Geometry: see drawing. Coordinates: mm, zero at the bounding-box minimum. A direction names the side the tool comes from. Coordinates: 2 decimals unless noted, no trailing zeros. Write each loop counter-clockwise with the first axis right and the second up, starting at its lowest first coordinate (ties: lowest second). Pieces come first, ordered by that corner, then holes. Notation, with made-up numbers: (-1.5, 39) -> (55.5, 39) arc R18 ccw to (55.5, 47) -> close; hole circle Ø1 at (29.25, 68.5). An arc over 180 degrees is marked (long way). Answer as a JSON object with one key per item and string values. Group by question number.
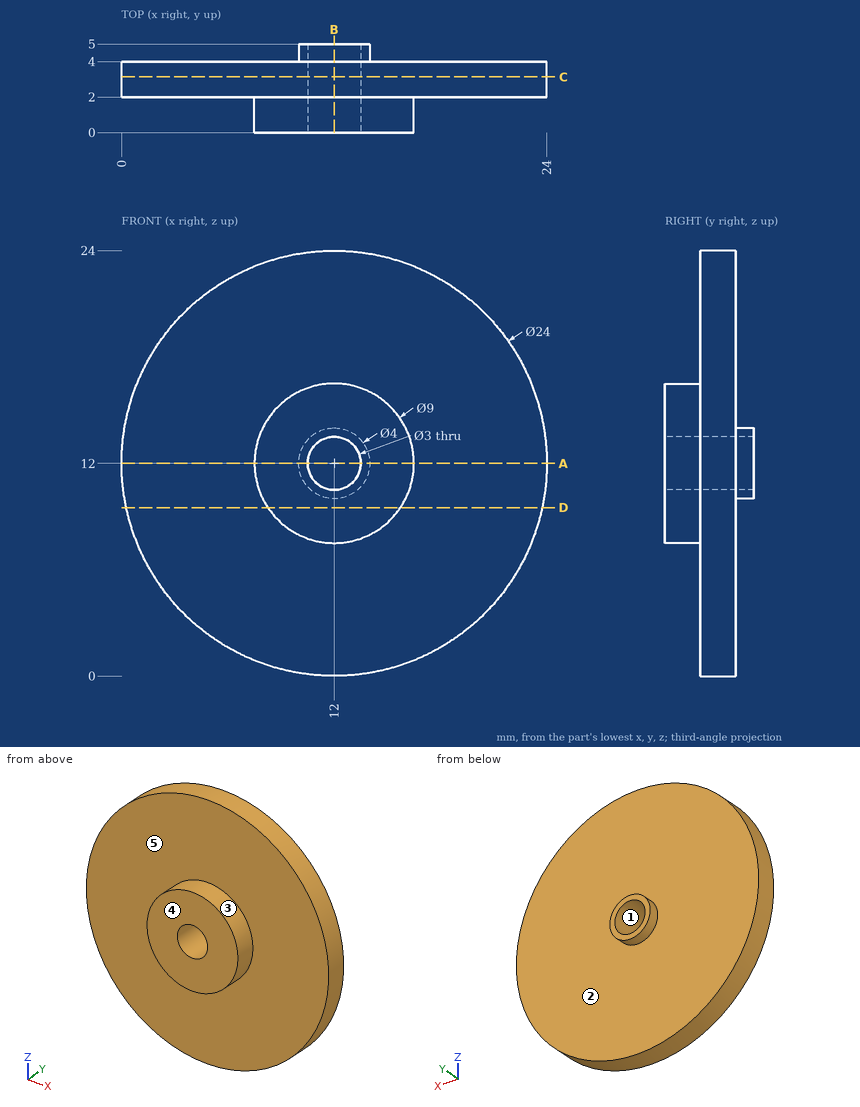
Item 1: Section B-B on x = 12. Output: boundary loops of the cut face in (y, z).
Item 2: Section A-A on z = 12. Output: boundary loops of the cut face in (x, y).
Item 3: Section C-C on y = 3.15. Output: boundary loops of the cut face in (x, z).
Item 4: Set-up query: the marked faces 4 and 5. Return all of +Z, -Z, +X, -X, +Y, -Y with unobstructed straight access to the full face (end or side cutting, diameter ignored); none if empty.
Item 5: Contact query for flat-ended pins moving along their axis: pin 1 (3 mm diameter, centred on x = 4.5, z = 20, fed in from +Y); pin 2 (2 mm diameter, centred on x = 5, y = 1.5, fed in from +Z); pin 3 (4 mm diameter, centred on x = 21, z = 21.5, fed in from -Y). Output: stop coordinate, or through.
Item 6: Ray query, L1, parallel to X at y = 1.9, z = 12; L2, parallel to X at y = 3.7, z = 12; L3, parallel to Y at x = 18.75, z = 6.25. Return the intervals inside material, ascending. Write a range as [from, to].
Item 7: Mould query, pull axis X, two halves, no side actions, for the marked faces 1, 2 and 3. Classes: +X half, -X half, draft (parallel to the pull), parting line (faces both ways), or undercut.
Item 8: Section D-D on z = 9.5. Output: boundary loops of the cut face in (x, y), then the cut area to 3 significant figures.
Answer sheet:
{
 "1": {"outline": "(0, 7.5) -> (2, 7.5) -> (2, 0) -> (4, 0) -> (4, 10) -> (5, 10) -> (5, 10.5) -> (0, 10.5) -> close; (0, 13.5) -> (5, 13.5) -> (5, 14) -> (4, 14) -> (4, 24) -> (2, 24) -> (2, 16.5) -> (0, 16.5) -> close"},
 "2": {"outline": "(0, 2) -> (7.5, 2) -> (7.5, 0) -> (10.5, 0) -> (10.5, 5) -> (10, 5) -> (10, 4) -> (0, 4) -> close; (13.5, 0) -> (16.5, 0) -> (16.5, 2) -> (24, 2) -> (24, 4) -> (14, 4) -> (14, 5) -> (13.5, 5) -> close"},
 "3": {"outline": "circle Ø24 at (12, 12); hole circle Ø3 at (12, 12)"},
 "4": {"face 4": "+Z, -Z, +X, -X, -Y", "face 5": "-Y"},
 "5": {"pin 1": "stops at y = 4", "pin 2": "stops at z = 22.31", "pin 3": "stops at y = 2"},
 "6": {"L1": "x = [7.5, 10.5], [13.5, 16.5]", "L2": "x = [0, 10.5], [13.5, 24]", "L3": "y = [2, 4]"},
 "7": {"face 1": "undercut", "face 2": "draft", "face 3": "parting line"},
 "8": {"outline": "(0.26, 2) -> (8.26, 2) -> (8.26, 0) -> (15.74, 0) -> (15.74, 2) -> (23.74, 2) -> (23.74, 4) -> (0.26, 4) -> close", "area": "61.9 mm^2"}
}
